Input: dimensioned drawing with shaded views. Units: mm. Origin: part minimum x, y, z. Round coordinates to 2 decimals unless told otherwise and drop trailing zeros. Loops run counter-clockwise (first coordinate to the right, second up) from the corner with the lowest first, then second, coordinate; pieces in that order, holes last. Notation, with made-up numbers: (-32, -19) - (16, -19) arc R28 ccw to (16, 20) - close; hole circle Ø2 at (69.25, 26). An arc over 180 degrees is marked (long way). Answer as a JSON object with one key per item and string values. Group by question number.
Item 1: Section C-C (x = 8). Return the cut outline in (y, z).
Item 2: Line query: line 1 (X direction, y = 2.7, z = 6.5); line 2 (X direction, y = 1.2, z = 8); line 3 (Y direction, x = 14.5, z = 6.5). Output: solid intervals per line, ascending.
Item 3: Draft query along X for the marked faces 1, 2, 3 and 4. Return one class per face: released by +X, released by -X, zero draft, split by the parting line, or undercut.
Item 4: Section D-D (z = 2.5). Count the separate pieces of the cut face and the enclosed holes in it, plus the area to 3 significant figures.
Item 5: First-contact query: pin 1 (0.8 mm diameter, centred on x = 25.5, y = 2.5, fed in from -Z); pin 2 (0.8 mm diameter, centred on y = 0.5, z = 1.5, fed in from +X); pin 3 (1.6 mm diameter, centred on x = 18.4, z = 2.5, fed in from -Y); pin 4 (1.5 mm diameter, centred on x = 16.5, y = 1.5, fed in from +Z). Flat tips, straight axial feed; report the tip coordinate or a pass-through.
Item 6: Section B-B (z = 10). Return the cut outline in (x, y).
Item 7: Section A-A (y = 1.3). Return the cut outline in (x, z), plus the area to 3 significant figures.
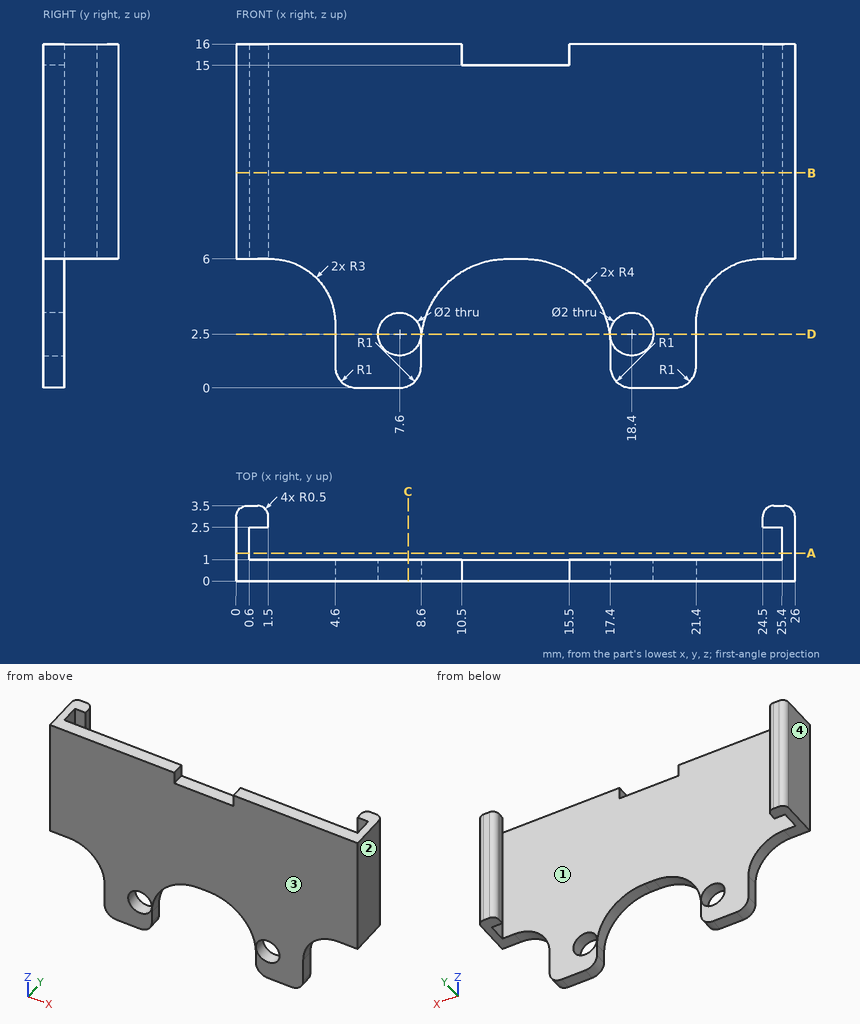
Values:
{
 "1": {"outline": "(0, 0.08) - (1, 0.08) - (1, 1.58) - (0, 1.58) - close; (0, 3.42) - (1, 3.42) - (1, 16) - (0, 16) - close"},
 "2": {"line 1": "x = 0 to 1.5, 24.5 to 26", "line 2": "x = 0 to 0.6, 25.4 to 26", "line 3": "y = 0 to 1"},
 "3": {"face 1": "undercut", "face 2": "released by +X", "face 3": "zero draft", "face 4": "released by -X"},
 "4": {"separate pieces": "4", "enclosed holes": "0", "area": "4.06 mm^2"},
 "5": {"pin 1": "stops at z = 6", "pin 2": "stops at x = 21.4", "pin 3": "passes through", "pin 4": "stops at z = 16"},
 "6": {"outline": "(0, 0) - (26, 0) - (26, 3) arc R0.5 ccw to (25.5, 3.5) - (25, 3.5) arc R0.5 ccw to (24.5, 3) - (24.5, 2.5) - (25.4, 2.5) - (25.4, 1) - (0.6, 1) - (0.6, 2.5) - (1.5, 2.5) - (1.5, 3) arc R0.5 ccw to (1, 3.5) - (0.5, 3.5) arc R0.5 ccw to (0, 3) - close"},
 "7": {"outline": "(0, 6) - (0.6, 6) - (0.6, 16) - (0, 16) - close; (25.4, 6) - (26, 6) - (26, 16) - (25.4, 16) - close", "area": "12.0 mm^2"}
}
